Part print with two shaded views. Sizes in mm from the minimum x, y, z corner. A direction names the side the tool comes from. Coordinates: 2 decimals unless noted, no trailing zeros. Order: outer loops, then holes, each group sorted by start corner. A loop starts at its lowest first (then second) coordinate and runs counter-clockwise, first axis right, second up. Notation, with made-up numbers: (74, -31) - (108, -31) arc R15 cw to (108, -8) - close; hole circle Ø4 at (22, -14.5). An arc over 180 degrees is marked (long way). One line per item, written item: value.
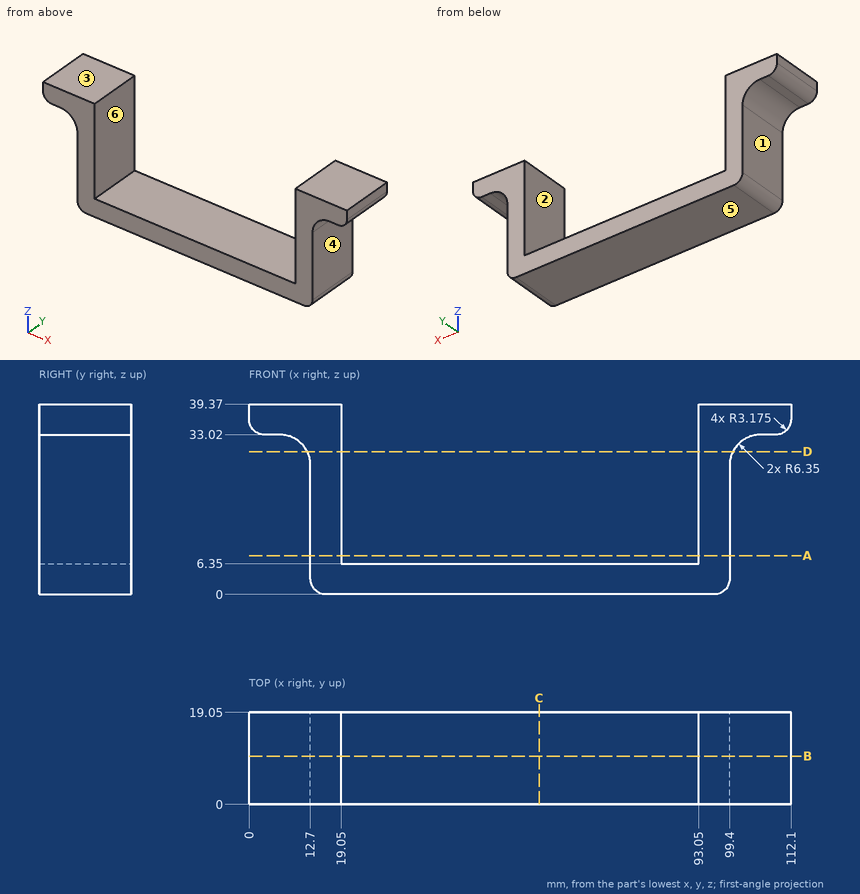
1. Probe line 1 along X through (y, z) = (4.75, 23); line 2 along Z through (x, y) = (35, 3); line 3 along X through (y, z) = (15.75, 38.5). List the from-to ranges inside material, lowest first.
Values found:
line 1: x = 12.7 to 19.05, 93.05 to 99.4
line 2: z = 0 to 6.35
line 3: x = 0 to 19.05, 93.05 to 112.1
2. Two-plate mould, pull along X, no slides. Class the marked faces 1, 2 and 3: pulls with the +X half, pulls with the -X half, needs draft (parallel to the pull), parting line crosses it, or undercut.
Values found:
face 1: pulls with the -X half
face 2: undercut
face 3: needs draft
3. Flat gauge pins, fed straight in: P1, Ø6, axis at y = 14.5, z = 7, coming from the -X side; P2, Ø5.5, axis at y = 13, z = 30.5, coming from the +X side; P3, Ø1, axis at x = 5, y = 9.5, coming from the -Z side. Where does each tip first touch, or does it go through?
Values found:
P1: stops at x = 12.7
P2: stops at x = 110.11
P3: stops at z = 33.02
4. Band-saw the part on B-B, the plane y = 10. Give the cut face in (x, z) (3 decimals).
Values found:
outline: (0, 36.195) arc R3.175 ccw to (3.175, 33.02) - (6.35, 33.02) arc R6.35 cw to (12.7, 26.67) - (12.7, 3.175) arc R3.175 ccw to (15.875, 0) - (96.225, 0) arc R3.175 ccw to (99.4, 3.175) - (99.4, 26.67) arc R6.35 cw to (105.75, 33.02) - (108.925, 33.02) arc R3.175 ccw to (112.1, 36.195) - (112.1, 39.37) - (93.05, 39.37) - (93.05, 6.35) - (19.05, 6.35) - (19.05, 39.37) - (0, 39.37) - close
5. Band-saw the part on A-A, the plane z = 8. Give the cut face in (x, y).
Values found:
outline: (12.7, 0) - (19.05, 0) - (19.05, 19.05) - (12.7, 19.05) - close; (93.05, 0) - (99.4, 0) - (99.4, 19.05) - (93.05, 19.05) - close
6. Band-saw the part on C-C, the plane x = 60. Give the cut face in (y, z).
Values found:
outline: (0, 0) - (19.05, 0) - (19.05, 6.35) - (0, 6.35) - close
7. 3-axis set-ups, long thin cutter, end or side, ignore diameter. For the marked faces 4, 5 and 6: which of +Z, -Z, +X, -X, +Y, -Y reach the whole face in a straight line?
Values found:
face 4: -Z, +X, +Y, -Y
face 5: -Z, +X, -X, +Y, -Y
face 6: +Z, +Y, -Y
8. Band-saw the part on D-D, the plane z = 29.5. Give the cut face in (x, y).
Values found:
outline: (12.03, 0) - (19.05, 0) - (19.05, 19.05) - (12.03, 19.05) - close; (93.05, 0) - (100.07, 0) - (100.07, 19.05) - (93.05, 19.05) - close
